Part model, mm, in its own coordinate system. A direction names the side the tool comes from. Round coordinates to 2 decimals unless told otherwise and drop trailing zeros. Order: outer loops, then holes, each group sorted by start corner. A loop starts at its lowest first (then second) coordinate and runs counter-clockwise, first axis right, second up. Notation, with made-up numbers: (74.5, 53) - (123.5, 53) arc R14 cw to (123.5, 78) - close; hole circle Ø4 at (58.5, 89.25). An arc over 180 degrees is marked (long way). Answer as a JSON object with one key per item and string values.
```python
from build123d import *

# Parameters (mm, degrees)
F0_R     = 20.6375
F1_DEPTH = 25.4
F0_W     = 82.55
F0_H     = 19.05
F2_DEPTH = 190.5
F3_R     = 17.4625
F4_DEPTH = 25.4


with BuildPart() as f1:
    # F0 (on Right) → F1 (new body)
    with BuildSketch(Plane.YZ):
        with BuildLine():
            Line((0, 57.15), (0, 19.05))
            Line((0, 19.05), (82.55, 19.05))
            Line((82.55, 19.05), (82.55, 57.15))
            ThreePointArc((82.55, 57.15), (41.275, 98.425), (0, 57.15))
        make_face()
        with Locations((41.275, 57.15)):
            Circle(F0_R, mode=Mode.SUBTRACT)
    extrude(amount=F1_DEPTH)

    # F0 (on Right) → F2 (join)
    with BuildSketch(Plane.YZ):
        with Locations((41.275, 9.525)):
            Rectangle(F0_W, F0_H)
    extrude(amount=F2_DEPTH)

    # F3 (on face) → F4 (cut)
    with BuildSketch(Plane.XY.offset(19.05)):
        with Locations((76.2, 41.179956)):
            Circle(F3_R)
        with Locations((152.4, 41.179956)):
            Circle(F3_R)
    extrude(amount=-F4_DEPTH, mode=Mode.SUBTRACT)


solid = f1.part
```
Item 1: Cut at A-A (x = 76.2). Write the cut outline in (y, z), plus the area to 3 significant figures.
Taken from the geometry:
{"outline": "(0, 0) - (23.72, 0) - (23.72, 19.05) - (0, 19.05) - close; (58.64, 0) - (82.55, 0) - (82.55, 19.05) - (58.64, 19.05) - close", "area": "907 mm2"}
Item 2: Probe L1, parallel to Y at x = 76.2, z = 4.75; L2, parallel to Y at x = 13, z = 57; L3, parallel to X at y = 26.5, z = 6. List the from-to ranges inside material, lowest first. Write a range as from..to.
Taken from the geometry:
{"L1": "0..23.72, 58.64..82.55", "L2": "0..20.64, 61.91..82.55", "L3": "0..66.74, 85.66..142.94, 161.86..190.5"}
Item 3: Two-plate mould, pull along Y, no slides. Class faces 3 (the cylindrical face through (92.33, 34.49, 9.66)), 4 (the flat face through (107, 41, 19.05)), 5 (the flat face through (73, 0, 15)): pulls with the +Y half, pulls with the -Y half, needs draft (parallel to the pull), parting line crosses it, or undercut.
Taken from the geometry:
{"face 3": "undercut", "face 4": "needs draft", "face 5": "pulls with the -Y half"}
Item 4: Drop flat-ended pins along their axis: P1, Ø12, axis at x = 33, y = 15.5, coming from the +Z side; P2, Ø1, axis at y = 18.5, z = 69, coming from the -X side. Give the stop position or say it passes through.
Taken from the geometry:
{"P1": "z = 19.05", "P2": "x = 0"}
Item 5: Cut at C-C (y = 49). Write the cut outline in (x, z).
Taken from the geometry:
{"outline": "(0, 0) - (60.59, 0) - (60.59, 19.05) - (25.4, 19.05) - (25.4, 38.01) - (0, 38.01) - close; (0, 76.29) - (25.4, 76.29) - (25.4, 97.7) - (0, 97.7) - close; (91.81, 0) - (136.79, 0) - (136.79, 19.05) - (91.81, 19.05) - close; (168.01, 0) - (190.5, 0) - (190.5, 19.05) - (168.01, 19.05) - close"}
Item 6: Cut at D-D (z = 34.5). Write the cut outline in (x, y), plus the area to 3 significant figures.
Taken from the geometry:
{"outline": "(0, 0) - (25.4, 0) - (25.4, 82.55) - (0, 82.55) - close", "area": "2,100 mm2"}
Item 7: Tool access for faces 1 (the cylindrical face through (12.522, 38.588, 77.612)), 2 (the flat face through (25.4, 59, 68.1)): list every direction of +Z, -Z, +X, -X, +Y, -Y with a clear straight run to the whole face (end or side of a thin tool).
Taken from the geometry:
{"face 1": "+X, -X", "face 2": "+Z, +X, +Y, -Y"}
Item 8: Cut at B-B (z = 68.5). Write the cut outline in (x, y).
Taken from the geometry:
{"outline": "(0, 1.59) - (25.4, 1.59) - (25.4, 24.04) - (0, 24.04) - close; (0, 58.51) - (25.4, 58.51) - (25.4, 80.96) - (0, 80.96) - close"}
